Model file for the job. Use its own axes, mm. Give positions to 0.01 mm unless a question says otherwise; leave off trailing zeros. Loops run counter-clockwise (first coordinate to the right, second up) from the corner with the lowest first, then second, coordinate; pieces in that order, holes last. Notation, with made-up numbers: (-6.75, -3) - (28.25, -3) arc R9 ccw to (28.25, 5) - close; hole circle Ø10 at (80.5, 71.5). An arc over 180 degrees is marked (long way). Answer as CSV lines item,"result". Start each with the question number.
Item 1: Saw through at C-C on y = 55. Give the cut face in (x, z).
Item 2: Pin check, flat tips, straight feed: pin 1 (3 mm diameter, centred on x = 2, y = 90.5, fed in from -Z); pin 2 (1.5 mm diameter, centred on x = -1, y = 76, fed in from +Z); pin 3 (1.5 mm diameter, centred on x = 1, y = 55.5, fed in from +Z). Stop position of each tip, or through.
Item 3: Saw through at A-A on x = 1. Give the cut face in (y, z), plus the area to 3 significant figures.
Item 4: Drill centre lines: L1, parallel to Z at x = -1.75, y = 104; L2, parallel to Z at x = 0, y = 141; L3, parallel to Z at x = 0.25, y = 69. Where is each one in solid material? Low to high. Write a range as from..to.
Item 5: Saw through at B-B on z = 18. Give the cut face in (x, y).
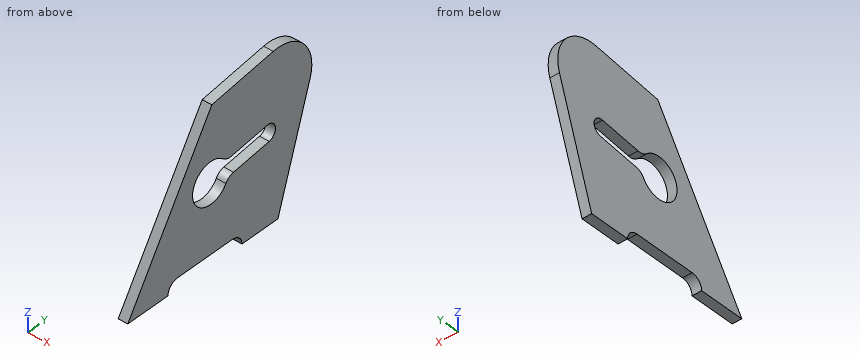
from build123d import *

# Parameters (mm, degrees)
BOSS_EXTRUDE1_DEPTH = 4
FILLET1_R           = 10


with BuildPart() as part:
    # Sketch1 → Boss-Extrude1 (new, symmetric)
    with BuildSketch(Plane.YZ):
        with BuildLine():
            Line((79.487889635, 127.207214423), (0, 0))
            Line((0, 0), (38, 0))
            ThreePointArc((38, 0), (40.636038969, 6.363961031), (47, 9))
            Line((47, 9), (99, 9))
            ThreePointArc((99, 9), (105.363961031, 6.363961031), (108, 0))
            Line((108, 0), (142, 0))
            Line((142, 0), (172.50354814, 93.880267937))
            ThreePointArc((172.50354814, 93.880267937), (166.569139078, 124.354715336), (137.573015724, 135.451290736))
            Line((137.573015724, 135.451290736), (79.487889635, 127.207214423))
        make_face()
        with BuildLine():
            ThreePointArc((94.543501955, 60.945796393), (61.402056741, 63.469750476), (92.64280616, 74.816173298))
            Line((92.64280616, 74.816173298), (131.785075785, 80.179945877))
            ThreePointArc((131.785075785, 80.179945877), (139.670612135, 74.195105322), (133.68577158, 66.309568971))
            Line((133.68577158, 66.309568971), (94.543501955, 60.945796393))
        make_face(mode=Mode.SUBTRACT)
    extrude(amount=BOSS_EXTRUDE1_DEPTH, both=True)

    # Fillet1
    fillet1_edges = [part.edges().sort_by_distance(p)[0] for p in [
        (0, 92.64280616, 74.816173298),
        (0, 94.543501955, 60.945796393),
    ]]
    fillet(fillet1_edges, radius=FILLET1_R)


solid = part.part
Responses:
1,outline,"(-4, 9) - (4, 9) - (4, 88.02) - (-4, 88.02) - close"
2,pin 1,"z = 9"
2,pin 2,"z = 122.83"
2,pin 3,"z = 90.02"
3,outline,"(0, 0) - (38, 0) arc R9 cw to (47, 9) - (99, 9) arc R9 cw to (108, 0) - (142, 0) - (172.5, 93.88) arc R32 ccw to (137.57, 135.45) - (79.49, 127.21) - close; hole (89.88, 78.18) arc R17 ccw (long way) to (92.78, 56.97) arc R10 cw to (99.98, 61.69) - (133.69, 66.31) arc R7 ccw to (131.79, 80.18) - (98.08, 75.56) arc R10 cw to start"
3,area,"13,700 mm2"
4,L1,"7.48..62.24, 76.37..130.69"
4,L2,"0..135.75"
4,L3,"9..51.51, 80.04..110.42"
5,outline,"(-4, 11.25) - (4, 11.25) - (4, 147.85) - (-4, 147.85) - close"
